```python
from build123d import *

# Parameters (mm, degrees)
PAD_DEPTH       = 15
SKETCH001_R     = 4.3
POCKET_DEPTH    = 60.001
SKETCH002_R     = 6.75
POCKET001_DEPTH = 55.001
FILLET_R        = 4
FILLET001_R     = 18
POCKET002_DEPTH = 3
GROOVE_ANGLE    = 90
FILLET002_R     = 3


with BuildPart() as part:
    # Sketch → Pad (new body)
    with BuildSketch(Plane.XZ):
        with BuildLine():
            ThreePointArc((-40.4, 46.4), (-30.500505, 50.500505), (-26.4, 60.4))
            Line((-26.4, 60.4), (26.4, 60.4))
            ThreePointArc((26.4, 60.4), (30.500505, 50.500505), (40.4, 46.4))
            Line((40.4, 5.4), (40.4, 46.4))
            Line((65.4, 5.4), (40.4, 5.4))
            Line((65.4, 15.4), (65.4, 5.4))
            Line((34.553176, 65.4), (65.4, 15.4))
            Line((-34.553176, 65.4), (34.553176, 65.4))
            Line((-65.4, 15.4), (-34.553176, 65.4))
            Line((-65.4, 5.4), (-65.4, 15.4))
            Line((-40.4, 5.4), (-65.4, 5.4))
            Line((-40.4, 46.4), (-40.4, 5.4))
        make_face()
    extrude(amount=PAD_DEPTH)

    # Sketch001 (on Face11 of Pad) → Pocket (cut, through all)
    with BuildSketch(Plane(origin=(0, 0, 5.4), x_dir=(1, 0, 0), z_dir=(0, 0, -1))):
        with Locations((-52.9, 7.5)):
            Circle(SKETCH001_R)
        with Locations((52.9, 7.5)):
            Circle(SKETCH001_R)
    extrude(amount=-POCKET_DEPTH, mode=Mode.SUBTRACT)

    # Sketch002 (on Face6 of Pocket) → Pocket001 (cut, through all)
    with BuildSketch(Plane(origin=(0, 0, 10.4), x_dir=(1, 0, 0), z_dir=(0, 0, -1))):
        with Locations((-52.9, 7.5)):
            Circle(SKETCH002_R)
        with Locations((52.9, 7.5)):
            Circle(SKETCH002_R)
    extrude(amount=-POCKET001_DEPTH, mode=Mode.SUBTRACT)

    # Fillet
    fillet_edges = [part.edges().sort_by_distance(p)[0] for p in [
        (-65.4, -15, 10.4),
        (-65.4, 0, 10.4),
        (65.4, -15, 10.4),
        (65.4, 0, 10.4),
    ]]
    fillet(fillet_edges, radius=FILLET_R)

    # Fillet001
    fillet001_edges = [part.edges().sort_by_distance(p)[0] for p in [
        (-34.553176, -7.5, 65.4),
        (34.553176, -7.5, 65.4),
    ]]
    fillet(fillet001_edges, radius=FILLET001_R)

    # Sketch003 (on Face16 of Fillet001) → Pocket002 (cut)
    with BuildSketch(Plane.XZ.offset(15)):
        with BuildLine():
            ThreePointArc((-10, 65.4), (-9.12132, 63.27868), (-7, 62.4))
            Line((-7, 62.4), (7, 62.4))
            ThreePointArc((7, 62.4), (9.12132, 63.27868), (10, 65.4))
            Line((-10, 65.4), (10, 65.4))
        make_face()
    extrude(amount=-POCKET002_DEPTH, mode=Mode.SUBTRACT)

    # Pocket002 Face21 → Groove (revolve, cut)
    with BuildSketch(Plane(origin=(0, -12, 63.957106), x_dir=(-1, 0, 0), z_dir=(0, -1, 0))):
        with BuildLine():
            ThreePointArc((10, -1.442894), (9.12132, 0.678426), (7, 1.557106))
            Line((7, 1.557106), (-7, 1.557106))
            ThreePointArc((-7, 1.557106), (-9.12132, 0.678426), (-10, -1.442894))
            Line((-10, -1.442894), (10, -1.442894))
        make_face()
    revolve(axis=Axis((0, -12, 65.4), (1, 0, 0)), revolution_arc=GROOVE_ANGLE, mode=Mode.SUBTRACT)

    # Fillet002
    fillet002_edges = [part.edges().sort_by_distance(p)[0] for p in [
        (0, -9, 65.4),
    ]]
    fillet(fillet002_edges, radius=FILLET002_R)


solid = part.part
```
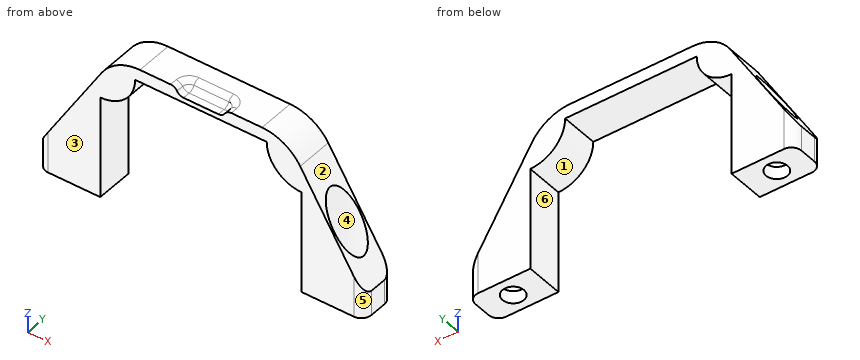
Build history of the part. All positions in model axes, mm. Face numbers are marked on the shaded views. A direction names the side the tool comes from. Round coordinates to 2 decimals unless told otherwise and drop trailing zeros. Loops run counter-clockwise (first coordinate to the right, second up) from the corner with the lowest first, then second, coordinate; pieces in that order, holes last.
Item 1: Saw through at C-C (z = 43). List the corners of the cut face in (x, y), then the cut area to 3 significant figures.
Item 2: Saw through at B-B (x = 0). List the corners of the cut face in (y, z), then the cut area to 3 significant figures.
Item 3: Drill centre lines: line 1 along X through (y, z) = (-7.5, 6.9); line 2 along Y through (x, z) = (52.9, 7.85); line 3 along X through (y, z) = (-9.25, 11.5). Where is each one in solid material? Low to high.
Item 4: Two-plate mould, pull along X, no slides. Class the marked faces 1, 2 and 3: released by +X, released by -X, zero draft, split by the parting line, or undercut.
Item 5: Saw through at A-A (z = 20). List the corners of the cut face in (x, y), then the cut area to 3 significant figures.
Item 6: Pin check, flat tips, straight feed: P1, Ø8, axis at y = -5.5, z = 38, coming from the +X side; P2, Ø1.5, axis at x = -3, y = -13.5, coming from the +Z side; P3, Ø7, axis at x = 52.5, y = -9.5, coming from the +Z side. Stop position of each tip, or through.
Item 7: Saw through at D-D (x = 50.5). List the corners of the cut face in (y, z).
Item 8: Which spindle directions (+Z, -Z, +X, -X, +Y, -Y) get a long thin tool onto all of the face, cutting with end or side? Do the marked faces 4, 5 and 6. Say none if no direction does.
Worked answers:
1. outline: (-48.37, -15) - (-40.4, -15) - (-40.4, 0) - (-48.37, 0) - (-48.37, -2.49) arc R6.75 cw to (-48.37, -12.51) - close; (40.4, -15) - (48.37, -15) - (48.37, -12.51) arc R6.75 cw to (48.37, -2.49) - (48.37, 0) - (40.4, 0) - close
1. area: 208 mm2
2. outline: (-15, 60.4) - (0, 60.4) - (0, 65.4) - (-6.8, 65.4) arc R3 ccw to (-9.4, 63.9) arc R3 cw to (-12, 62.4) - (-15, 62.4) - close
2. area: 58.2 mm2
3. line 1: x = -65.4 to -57.2, -48.6 to -40.4, 40.4 to 48.6, 57.2 to 65.4
3. line 2: y = -15 to -11.8, -3.2 to 0
3. line 3: x = -65.4 to -59.42, -46.38 to -40.4, 40.4 to 46.38, 59.42 to 65.4
4. face 1: undercut
4. face 2: released by +X
4. face 3: zero draft
5. outline: (-62.56, -14.83) arc R4 ccw to (-61.4, -15) - (-40.4, -15) - (-40.4, 0) - (-61.4, 0) arc R4 ccw to (-62.56, -0.17) - close; (40.4, -15) - (61.4, -15) arc R4 ccw to (62.56, -14.83) - (62.56, -0.17) arc R4 ccw to (61.4, 0) - (40.4, 0) - close; hole circle Ø13.5 at (-52.9, -7.5); hole circle Ø13.5 at (52.9, -7.5)
5. area: 378 mm2
6. P1: stops at x = 49.81
6. P2: stops at z = 62.4
6. P3: stops at z = 10.4
7. outline: (-15, 5.4) - (-11.07, 5.4) - (-11.07, 10.4) - (-13.81, 10.4) - (-13.81, 39.55) - (-15, 39.55) - close; (-3.93, 5.4) - (0, 5.4) - (0, 39.55) - (-1.19, 39.55) - (-1.19, 10.4) - (-3.93, 10.4) - close
8. face 4: +Z
8. face 5: +Z, -Z, +X, -Y
8. face 6: -Z, +Y, -Y
